Read the model definition and answer for the solid it produces. Units are mm, in the model's axes. Face numbers are marked on the shaded views. A direction names the side the tool comes from. Give positions to 0.01 mm unless a question says otherwise; leave off trailing zeros. Order: outer loops, then holes, each group sorted by start corner. A loop starts at its lowest first (then second) coordinate and runs counter-clockwise, first axis right, second up. Notation, with made-up numbers: (51, 66.5) -> (65, 66.5) arc R15 cw to (65, 87.5) -> close; hole circle Ø3 at (-2, 36). An arc over 180 degrees is marked (long way). One line per item, written item: value. Start each with the question number.
from build123d import *

# Parameters (mm, degrees)
SKETCH001_R          = 2.9845
POCKET_DEPTH         = 5.588
SKETCH002_R          = 0.7874
POCKET001_DEPTH      = 16.851
SKETCH004_W          = 0.5
SKETCH004_H          = 12.688059
SKETCH004_H_2        = 6.122161
POCKET003_DEPTH      = 5.0038
POCKET003_DEPTH_BACK = -5.0038
SKETCH005_W          = 1.27
SKETCH005_H          = 12.7
POCKET004_DEPTH      = 25.4
POCKET004_DEPTH_BACK = -23.7998


with BuildPart() as part:
    # Sketch → Revolution (revolve)
    with BuildSketch(Plane.XZ):
        Polygon((2.5, 0), (4, 0), (4, -6.35), (0, -6.35), (0, 0), (0, 10.5), (1.9, 10.5), (1.4, 9.15), (2.6, 3.5), (2.5, 2.5), align=None)
    revolve(axis=Axis((0, 0, 0), (0, 0, 1)))

    # Sketch001 (on Face5 of Revolution) → Pocket (cut)
    with BuildSketch(Plane(origin=(0, 0, -6.35), x_dir=(1, 0, 0), z_dir=(0, 0, -1))):
        Circle(SKETCH001_R)
    extrude(amount=-POCKET_DEPTH, mode=Mode.SUBTRACT)

    # Sketch002 (on Face6 of Pocket) → Pocket001 (cut, through all)
    with BuildSketch(Plane(origin=(0, 0, 10.5), x_dir=(-1, 0, 0), z_dir=(0, 0, 1))):
        Circle(SKETCH002_R)
    extrude(amount=-POCKET001_DEPTH, mode=Mode.SUBTRACT)

    # Sketch004 → Pocket003 (cut, two sides)
    with BuildSketch(Plane.XZ) as pocket003_sk:
        with Locations((0, 6.598029)):
            Rectangle(SKETCH004_W, SKETCH004_H)
        with Locations((0, -13.475635)):
            Rectangle(SKETCH004_W, SKETCH004_H_2)
    extrude(amount=-POCKET003_DEPTH, mode=Mode.SUBTRACT)
    extrude(pocket003_sk.sketch, amount=-POCKET003_DEPTH_BACK, mode=Mode.SUBTRACT)

    # Sketch005 → Pocket004 (cut, two sides)
    with BuildSketch(Plane.XZ) as pocket004_sk:
        with Locations((0, -8.89)):
            Rectangle(SKETCH005_W, SKETCH005_H)
    extrude(amount=-POCKET004_DEPTH, mode=Mode.SUBTRACT)
    extrude(pocket004_sk.sketch, amount=-POCKET004_DEPTH_BACK, mode=Mode.SUBTRACT)


solid = part.part
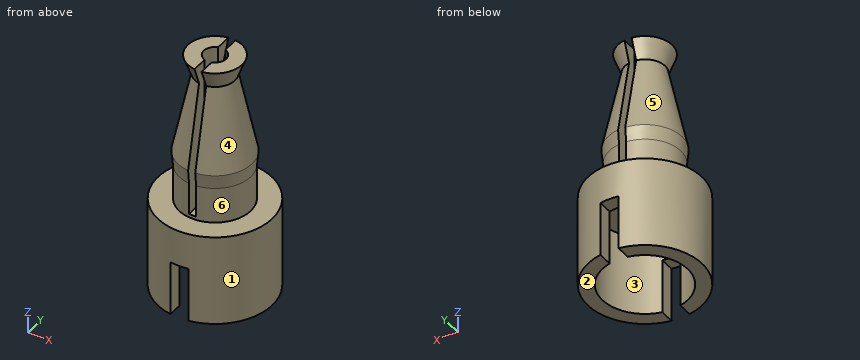
Item 1: Find section C-C on z = 2.25. Write down the section's boundary in (x, y), then the cut area to 3 significant figures.
Item 2: Find the intervals of material crossed by line 1 (X direction, y = 0, z = 2.25); line 2 (X direction, y = 0, z = -2.8), in increasing order. Write a range as from..to.
Item 3: Find section D-D on z = -1.75. Write down the section's boundary in (x, y), then the cut area to 3 significant figures.
Item 4: Find section A-A on x = 0. Write down the section's boundary in (y, z).
Item 5: For a pull along Y with two mould halves and no side action, classify the marked faces 1, 2 and 3 as +Y half, -Y half, draft (parallel to the pull), parting line (faces both ways), or undercut.
Item 6: Flat-ended cylindrical pins translate along their axes: pin 1 (0.8 mm diameter, centred on y = -3.5, z = -5, fed in from -X); pin 2 (1 mm diameter, centred on y = -1.5, z = 6.5, fed in from -X); pin 3 (0.8 mm diameter, centred on y = -3.5, z = -4.5, fed in from +X); pin 4 (0.6 mm diameter, centred on y = 2, z = 8, fed in from -X). Find the tip coordinate at first contact, or state that the pin passes through.
Item 7: A tool of negligible diameter and unlimited length cuts with its end or side. For the marked faces 4, 5 and 6, from which of +Z, -Z, +X, -X, +Y, -Y can it reach the whole face along a straight path? Write none if from no direction.
Item 8: Find section B-B on y = 0. Write down the section's boundary in (x, z).
Checks:
1. outline: (-0.25, -2.49) -> (-0.25, -0.75) arc R0.79 cw to (-0.25, 0.75) -> (-0.25, 2.49) arc R2.5 ccw to start; (0.25, -2.49) arc R2.5 ccw to (0.25, 2.49) -> (0.25, 0.75) arc R0.79 cw to (0.25, -0.75) -> close
1. area: 16.0 mm2
2. line 1: -2.5..-0.79, 0.79..2.5
2. line 2: -4..-2.98, 2.98..4
3. outline: circle Ø8 at (0, 0); hole circle Ø5.97 at (0, 0)
3. area: 22.3 mm2
4. outline: (-4, -2.54) -> (-2.98, -2.54) -> (-2.98, -0.76) -> (-0.79, -0.76) -> (-0.79, 0.25) -> (-2.5, 0.25) -> (-2.5, 0) -> (-4, 0) -> close; (0.79, -0.76) -> (2.98, -0.76) -> (2.98, -2.54) -> (4, -2.54) -> (4, 0) -> (2.5, 0) -> (2.5, 0.25) -> (0.79, 0.25) -> close
5. face 1: parting line
5. face 2: draft
5. face 3: undercut
6. pin 1: x = -2.53
6. pin 2: x = -1.71
6. pin 3: x = 2.53
6. pin 4: through
7. face 4: +X
7. face 5: -X
7. face 6: none
8. outline: (-4, -6.35) -> (-2.98, -6.35) -> (-2.98, -0.76) -> (-0.79, -0.76) -> (-0.79, 10.5) -> (-1.9, 10.5) -> (-1.4, 9.15) -> (-2.6, 3.5) -> (-2.5, 2.5) -> (-2.5, 0) -> (-4, 0) -> close; (0.79, -0.76) -> (2.98, -0.76) -> (2.98, -6.35) -> (4, -6.35) -> (4, 0) -> (2.5, 0) -> (2.5, 2.5) -> (2.6, 3.5) -> (1.4, 9.15) -> (1.9, 10.5) -> (0.79, 10.5) -> close
